Source: CAD feature listing. Evaluate the final solid. Frame: model axes, mm. A direction names the side the tool comes from. Round coordinates to 2 decimals unless told otherwise and drop trailing zeros. Loops run counter-clockwise (first coordinate to the right, second up) from the corner with the lowest first, then second, coordinate; pieces in that order, holes last.
Item 1: Pull-direction query (Z, two-part tool) for faces 3 (the flat face through (0, -4, -30)), 4 (the flat face through (0, -4, 25)), 5 (the flat face through (0, -4, 30)), 6 (the flat face through (0, 250, 27)); classes: released by +Z, released by -Z, zero draft, split by the parting line, or undercut.
Item 2: Section query C-C on y = -30. Return loops of the section in (x, z), then the cut area to 3 significant figures.
Item 3: Section query A-A on x = 23.5. Return loops of the section in (y, z).
Item 4: First-contact query: P1, Ø13.5, axis at x = 7.75, y = -163.58, coming from the -Z side. Flat tip, straight axial feed; report the tip coordinate or a pass-through.
Item 5: Section query B-B on z = 6.5. Return loops of the section in (x, y), then the cut area to 3 significant figures.
Item 6: Ray query, L1, parallel to Z at x = 6.5, y = 13.5; L2, parallel to X at y = 162.5, z = -5.5; L3, parallel to Y at x = 34.5, z = -24.5. Return the intervals inside material, ascending.
Item 7: Access query for faces 1 (the flat face through (0, -246, -25)), 2 (the cylindrical face through (-5.87, -55.28, 27.47)). Directions: +Z, -Z, +X, -X, +Y, -Y. A direction counts if a zero-diameter tool reaches every point of the face in a straight line with its end or side. Return the directions, or none.
```python
from build123d import *

# Parameters (mm, degrees)
F1_DEPTH = 250
F4_D     = 10.5
F6_D     = 10.5


with BuildPart() as f1:
    # F0 (on Front) → F1 (new body, symmetric)
    with BuildSketch(Plane.XZ):
        with BuildLine():
            ThreePointArc((40, 23), (37.9497474683, 27.9497474683), (33, 30))
            Line((33, 30), (-33, 30))
            ThreePointArc((-33, 30), (-37.9497474683, 27.9497474683), (-40, 23))
            Line((-40, 23), (-40, -23))
            ThreePointArc((-40, -23), (-37.9497474683, -27.9497474683), (-33, -30))
            Line((-33, -30), (33, -30))
            ThreePointArc((33, -30), (37.9497474683, -27.9497474683), (40, -23))
            Line((40, -23), (40, 23))
        make_face()
        with BuildLine():
            Line((-33, 25), (33, 25))
            ThreePointArc((33, 25), (34.4142135624, 24.4142135624), (35, 23))
            Line((35, 23), (35, -23))
            ThreePointArc((35, -23), (34.4142135624, -24.4142135624), (33, -25))
            Line((33, -25), (-33, -25))
            ThreePointArc((-33, -25), (-34.4142135624, -24.4142135624), (-35, -23))
            Line((-35, -23), (-35, 23))
            ThreePointArc((-35, 23), (-34.4142135624, 24.4142135624), (-33, 25))
        make_face(mode=Mode.SUBTRACT)
    extrude(amount=F1_DEPTH, both=True)

    # F4 (through all)
    with Locations(Plane.XY.offset(30)):
        with Locations((7.7468804084, -163.5783314705), (-6.5550529398, -60.4852437973), (8.3427932113, 82.5340524316), (4.7673056833, 151.0641425848), (-16.68558456, 199.3331462145)):
            Hole(F4_D / 2)

    # F6 (through all)
    with Locations(Plane.YZ.offset(40)):
        with Locations((-240, -20)):
            Hole(F6_D / 2)


solid = f1.part
```
Data:
1. face 3: released by -Z
1. face 4: undercut
1. face 5: released by +Z
1. face 6: zero draft
2. outline: (-40, -23) arc R7 ccw to (-33, -30) - (33, -30) arc R7 ccw to (40, -23) - (40, 23) arc R7 ccw to (33, 30) - (-33, 30) arc R7 ccw to (-40, 23) - close; hole (-35, -23) arc R2 ccw to (-33, -25) - (33, -25) arc R2 ccw to (35, -23) - (35, 23) arc R2 ccw to (33, 25) - (-33, 25) arc R2 ccw to (-35, 23) - close
2. area: 1,260 mm2
3. outline: (-250, -30) - (250, -30) - (250, -25) - (-238.4, -25) arc R5.25 cw to (-241.6, -25) - (-250, -25) - close; (-250, 25) - (250, 25) - (250, 30) - (-250, 30) - close
4. P1: stops at z = -30
5. outline: (-40, -250) - (-35, -250) - (-35, 250) - (-40, 250) - close; (35, -250) - (40, -250) - (40, 250) - (35, 250) - close
5. area: 5,000 mm2
6. L1: z = -30 to -25, 25 to 30
6. L2: x = -40 to -35, 35 to 40
6. L3: y = -250 to -242.7, -237.3 to 250
7. face 1: +Y, -Y
7. face 2: +Z, -Z
